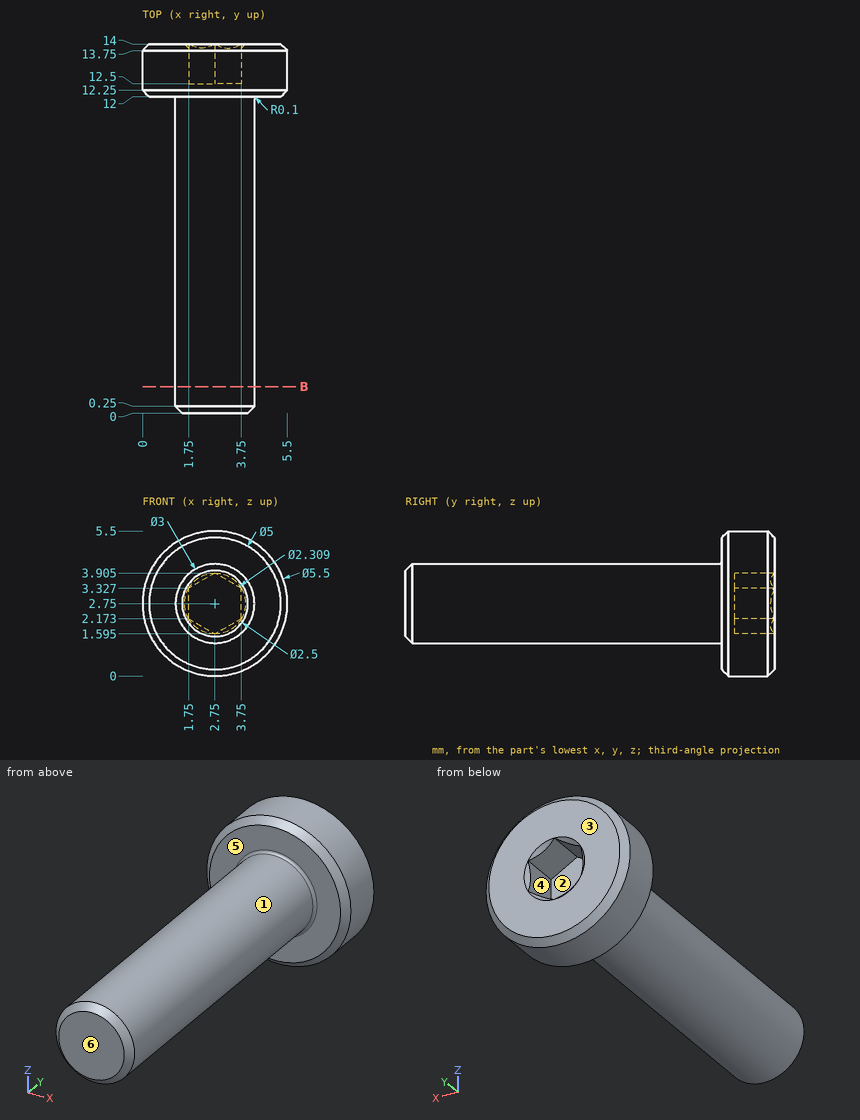
Geometry: see drawing. Coordinates: mm, zero at the bounding-box minimum. A direction names the side the tool comes from. Coordinates: 2 decimals unless noted, no trailing zeros. Loops run counter-clockwise (first coordinate to the right, second up) from the corner with the lowest first, then second, coordinate; pieces in that order, holes last. Notation, with made-up numbers: (-6, 86.25) -> (16, 86.25) arc R30 cw to (16, 109.25) -> close; hole circle Ø6 at (41, 48). An arc over 180 degrees is marked (long way). Use a Markdown table: item, result.
1) Pull-direction query (X, two-part tool) for the marked faces 1, 2 and 3; classes: released by +X, released by -X, zero draft, split by the parting line, or undercut.
Results found:
| item | result |
|---|---|
| face 1 | split by the parting line |
| face 2 | undercut |
| face 3 | zero draft |
2) Access query for the marked faces 4, 5 and 6. Directions: +Z, -Z, +X, -X, +Y, -Y. A direction counts if a zero-diameter tool reaches every point of the face in a straight line with its end or side. Return the directions, or none.
Results found:
| item | result |
|---|---|
| face 4 | +Y |
| face 5 | -Y |
| face 6 | +Z, -Z, +X, -X, -Y |
3) Material intervals for line 1 along X through (y, z) = (13, 2.8); line 2 along Y through (x, z) = (4.45, 2.7); line 3 along Y through (x, z) = (2.9, 3), sorted ascending. Write a range as from..to.
Results found:
| item | result |
|---|---|
| line 1 | x = 0..1.75, 3.75..5.5 |
| line 2 | y = 12..14 |
| line 3 | y = 0..12.5 |
4) Contact query for flat-ended pins moving along their axis: pin 1 (1 mm diameter, centred on x = 1, y = 8.5, fed in from -Z); pin 2 (1.5 mm diameter, centred on x = 3.5, y = 11, fed in from -Z); pin 3 (3 mm diameter, centred on y = 4, z = 2, fed in from +X). Output: stop coordinate, or through.
Results found:
| item | result |
|---|---|
| pin 1 | stops at z = 1.92 |
| pin 2 | stops at z = 1.25 |
| pin 3 | stops at x = 4.25 |
5) Cut plane B-B (y = 1). Return the cut outline in (x, z).
Results found:
| item | result |
|---|---|
| outline | circle Ø3 at (2.75, 2.75) |
